from build123d import *

# Parameters (mm, degrees)
SKETCH1_W           = 20
SKETCH1_H           = 9
BOSS_EXTRUDE1_DEPTH = 13
CUT_EXTRUDE1_DEPTH  = 3
FILLET1_R           = 3
SKETCH3_W           = 20
SKETCH3_H           = 4
CUT_EXTRUDE2_DEPTH  = 61
SKETCH3_3_W         = 20
SKETCH3_3_H         = 4
BOSS_EXTRUDE2_DEPTH = 13
FILLET4_R           = 1


with BuildPart() as part:
    # Sketch1 → Boss-Extrude1 (new body)
    with BuildSketch(Plane.XY):
        Rectangle(SKETCH1_W, SKETCH1_H)
    extrude(amount=BOSS_EXTRUDE1_DEPTH)

    # Sketch2 → Cut-Extrude1 (cut)
    with BuildSketch(Plane.XY.offset(13)):
        with BuildLine():
            Line((1.51, -4.5), (1.51, -4.099981132))
            ThreePointArc((1.51, -4.099981132), (0, 1.6), (-1.51, -4.099981132))
            Line((-1.51, -4.099981132), (-1.51, -4.5))
            Line((-1.51, -4.5), (1.51, -4.5))
        make_face()
    extrude(amount=-CUT_EXTRUDE1_DEPTH, mode=Mode.SUBTRACT)

    # Fillet1
    fillet1_edges = [part.edges().sort_by_distance(p)[0] for p in [
        (-10, 4.5, 6.5),
        (10, 4.5, 6.5),
    ]]
    fillet(fillet1_edges, radius=FILLET1_R)

    # Sketch3 → Cut-Extrude2 (cut)
    with BuildSketch(Plane.XZ.offset(4.5)):
        with Locations((0, 2)):
            Rectangle(SKETCH3_W, SKETCH3_H)
    extrude(amount=-CUT_EXTRUDE2_DEPTH, mode=Mode.SUBTRACT)

    # Sketch3<3> → Boss-Extrude2 (add)
    with BuildSketch(Plane.XZ.offset(4.5)):
        with Locations((0, 6)):
            Rectangle(SKETCH3_3_W, SKETCH3_3_H)
    extrude(amount=BOSS_EXTRUDE2_DEPTH)

    # Fillet4
    fillet4_edges = [part.edges().sort_by_distance(p)[0] for p in [
        (9.121320344, 3.621320344, 4),
        (0, 4.5, 4),
        (10, -8, 4),
        (-9.121320344, 3.621320344, 4),
        (-10, -8, 4),
    ]]
    fillet(fillet4_edges, radius=FILLET4_R)


solid = part.part
Design review of the part built by this model. Coordinates are the model's own, in mm. A direction names the side the tool comes from. Round coordinates to 2 decimals unless told otherwise and drop trailing zeros. Write each loop counter-clockwise with the first axis right and the second up, starting at its lowest first coordinate (ties: lowest second). Pieces come first, ordered by that corner, then holes.
Item 1: Consider section A-A on z = 12. Give the boundary of the cut face in (x, y), and give its area (3 significant figures).
Item 2: Consider section C-C on x = -4.5. Give the boundary of the cut face in (y, z), and give its area (3 significant figures).
Item 3: For pin 1 Ø1.8 at (x, y) = (1.5, -1.5) entering from +Z; pin 2 Ø2 at (y, z) = (-9, 8.5) entering from -X; pin 3 Ø10.5 at (x, y) = (4, -10.5) entering from +Z, all flat-tipped, find the tip position at first contact; note any pin that passes through.
Item 4: Draft analysis for pull direction X (two halves, no side actions). For faces 1 (the cylindrical face through (9.1, 3.64, 9.06)), 2 (the cylindrical face through (-9.14, 3.6, 9.06)), 3 (the flat face through (0, 2, 13)), 4 (the flat face through (0, -1, 10)), state which applies: released by +X, released by -X, zero draft, split by the parting line, or undercut.
Item 5: For faces 5 (the flat face through (0, 4.5, 9)), 6 (the cylindrical face through (0.1, 1.6, 11.5)), 7 (the flat face through (0, -11, 8)), list the 3-axis set-ups (+Z, -Z, +X, -X, +Y, -Y) from which the entire face can be reached by the end or side of a thin tool; tool diameter is ignored.
Item 6: Wall thickness on L1, parallel to X at y = -1.45, z = 11.65; L2, parallel to Y at x = -3.25, z = 11.25; L3, parallel to Y at x = 0, z = 11.85: over which ranges is each line inside the solid? List them lowest first.
Item 7: Consider section B-B on y = -13.75. Give the boundary of the cut face in (x, z).
Item 8: Consider section D-D on y = -1.45. Give the boundary of the cut face in (x, z).
Check values:
1. outline: (-10, -4.5) - (-1.51, -4.5) - (-1.51, -4.1) arc R3.05 cw (long way) to (1.51, -4.1) - (1.51, -4.5) - (10, -4.5) - (10, 1.5) arc R3 ccw to (7, 4.5) - (-7, 4.5) arc R3 ccw to (-10, 1.5) - close
1. area: 147 mm2
2. outline: (-17.5, 4) - (3.5, 4) arc R1 ccw to (4.5, 5) - (4.5, 13) - (-4.5, 13) - (-4.5, 8) - (-17.5, 8) - close
2. area: 133 mm2
3. pin 1: stops at z = 10
3. pin 2: stops at x = -10
3. pin 3: stops at z = 8
4. face 1: released by +X
4. face 2: released by -X
4. face 3: zero draft
4. face 4: undercut
5. face 5: +Z, -Z, +X, -X, +Y
5. face 6: +Z
5. face 7: +Z, +X, -X, -Y
6. L1: x = -10 to -3.05, 3.05 to 10
6. L2: y = -4.5 to 4.5
6. L3: y = 1.6 to 4.5
7. outline: (-10, 5) arc R1 ccw to (-9, 4) - (9, 4) arc R1 ccw to (10, 5) - (10, 8) - (-10, 8) - close
8. outline: (-10, 5) arc R1 ccw to (-9, 4) - (9, 4) arc R1 ccw to (10, 5) - (10, 13) - (3.05, 13) - (3.05, 10) - (-3.05, 10) - (-3.05, 13) - (-10, 13) - close
